The model under review builds one solid part; all positions refer to its coordinate system, in mm. A direction names the side the tool comes from. Give positions to 0.01 mm unless a question says otherwise; leave off trailing zeros. Write each loop counter-clockwise with the first axis right and the second up, starting at its lowest first coordinate (ties: lowest second). Pieces come first, ordered by that corner, then holes. Notation, with made-up numbers: M 60.25,12 L 80.25,12 A11 cw 80.25,17 Z; hole C 26.25,16.25 d1. An arc over 180 degrees is marked long. Write each question's results on one line, items separated by ' | '. Start each with the question number.
from build123d import *

# Parameters (mm, degrees)
VARREDURA1_PROFILE_R          = 2.3
ESBO_O18_W                    = 4.8
ESBO_O18_H                    = 4.8
RESSALTO_EXTRUS_O1_DEPTH      = 20
RESSALTO_EXTRUS_O1_DEPTH_BACK = 7


with BuildPart() as part:
    # Varredura1: sweep along a path in Esboço1
    with BuildLine(Plane.XY) as varredura1_path:
        ThreePointArc((-10, -10), (-2.928932188, -7.071067812), (0, 0))
        Line((0, 0), (0, 25))
        ThreePointArc((0, 25), (-2.928932188, 32.071067812), (-10, 35))
    # Varredura1 profile (on start of the path) → Varredura1 (sweep)
    with BuildSketch(Plane(origin=(-10, -10, 0), x_dir=(0, 1, 0), z_dir=(1, 0, 0))):
        Circle(VARREDURA1_PROFILE_R)
    sweep(path=varredura1_path.line)

    # Esboço18 → Ressalto-extrusão1 (add, two sides)
    with BuildSketch(Plane.ZY.offset(10)) as ressalto_extrus_o1_sk:
        with Locations((0, -10)):
            Rectangle(ESBO_O18_W, ESBO_O18_H)
    extrude(amount=RESSALTO_EXTRUS_O1_DEPTH)
    extrude(ressalto_extrus_o1_sk.sketch, amount=-RESSALTO_EXTRUS_O1_DEPTH_BACK)


solid = part.part
(1) Add section C-C (y = 11). State the section outline as (x, z) points, then the cut area to 3 significant figures.
(2) Add section A-A (z = 0). State the section outline as (x, y) points.
(3) Draft analysis for pull direction Y (two halves, no side actions). For faces 4 (the cylindrical face through (0.499, 12.675, -2.245)), 5 (the flat face through (-17, -10, 2.4)), 6 (the flat face through (-17, -12.4, 0)), state which applies: pulls with the +Y half, pulls with the -Y half, needs draft (parallel to the pull), parting line crosses it, or undercut.
(4) Machinability: for faces 1 (the flat face through (-30, -10, 0)), 2 (the flat face through (-10, 35, 0)), 3 (the flat face through (-3, -11, 0)), which of the approach directions +Z, -Z, +X, -X, +Y, -Y give a long, thin tool a straight path to every point of the face, cutting with its end or side? Answer none if there is none.
(5) Add section B-B (x = -16). State the section outline as (y, z) points, then the cut area to 3 significant figures.
(6) Wall thickness on L1, parallel to Y at x = -16.5, z = -0.75; L2, parallel to Y at x = -3.5, z = 1.55; L3, parallel to Y at x = -8.5, z = -0.3: over which ranges is each line inside the solid? List them lowest first.
(7) Clearance check with flat-ended pins moving along their axes: P1, Ø1, axis at y = 25, z = -2, coming from the -X side; P2, Ø8, axis at x = -8, y = 3, coming from the +Z side; P3, Ø1, axis at y = -1, z = -1.5, coming from the +X side; P4, Ø1.4, axis at y = 35, z = -1, coming from the -X side. State where each tip first meets the part, or that it passes through.
Calculated:
1) outline: C 0,0 d4.6 | area: 16.6 mm²
2) outline: M -30,-12.4 L -3,-12.4 L -3,-10.11 A12.3 ccw 2.3,0 L 2.3,25 A12.3 ccw -10,37.3 L -10,32.7 A7.7 cw -2.3,25 L -2.3,0 A7.7 cw -8.76,-7.6 L -30,-7.6 Z
3) face 4: undercut | face 5: needs draft | face 6: pulls with the -Y half
4) face 1: +Z, -Z, -X, +Y, -Y | face 2: +Z, -Z, -X, +Y | face 3: +X, -Y
5) outline: M -12.4,-2.4 L -7.6,-2.4 L -7.6,2.4 L -12.4,2.4 Z | area: 23.0 mm²
6) L1: y = -12.4 to -7.6 | L2: y = -12.4 to -5.16, 30.16 to 34.73 | L3: y = -12.4 to -7.57, 32.57 to 37.19
7) P1: stops at x = -1.74 | P2: passes through | P3: stops at x = 2.03 | P4: stops at x = -10
